```python
from build123d import *

# Parameters (mm, degrees)
SKETCH1_R           = 2.0701
BOSS_EXTRUDE1_DEPTH = 2.286


with BuildPart() as part:
    # Sketch1 → Boss-Extrude1 (new body)
    with BuildSketch(Plane.XY.offset(2.286)):
        with BuildLine():
            Line((-12.7, 3.956428413), (-12.7, -68.893532285))
            Line((-12.7, -68.893532285), (-10.706695129, -69.723))
            Line((-10.706695129, -69.723), (11.870532285, -69.723))
            Line((11.870532285, -69.723), (12.7, -67.729695129))
            Line((12.7, -67.729695129), (12.7, -38.505245425))
            ThreePointArc((12.7, -38.505245425), (14.659980102, -35.571927909), (18.12006403, -36.260181395))
            Line((18.12006403, -36.260181395), (38.820161129, -56.960278494))
            Line((38.820161129, -56.960278494), (40.813466, -57.789746209))
            Line((40.813466, -57.789746209), (56.780673371, -41.822538838))
            Line((56.780673371, -41.822538838), (57.610141086, -39.829233967))
            Line((57.610141086, -39.829233967), (6.081013492, 11.699893628))
            Line((6.081013492, 11.699893628), (4.087708621, 12.529361343))
            Line((4.087708621, 12.529361343), (-11.870532285, 5.949733284))
            Line((-11.870532285, 5.949733284), (-12.7, 3.956428413))
        make_face()
        with Locations((0, -63.5)):
            Circle(SKETCH1_R, mode=Mode.SUBTRACT)
        with Locations((35.921024484, -35.921024484)):
            Circle(SKETCH1_R, mode=Mode.SUBTRACT)
        with Locations((17.960512242, -17.960512242)):
            Circle(SKETCH1_R, mode=Mode.SUBTRACT)
        with Locations((0, -38.1)):
            Circle(SKETCH1_R, mode=Mode.SUBTRACT)
        with Locations((0, -12.7)):
            Circle(SKETCH1_R, mode=Mode.SUBTRACT)
        Circle(SKETCH1_R, mode=Mode.SUBTRACT)
        with Locations((8.980256121, -8.980256121)):
            Circle(SKETCH1_R, mode=Mode.SUBTRACT)
        with Locations((0, -25.4)):
            Circle(SKETCH1_R, mode=Mode.SUBTRACT)
        with Locations((0, -50.8)):
            Circle(SKETCH1_R, mode=Mode.SUBTRACT)
        with Locations((26.940768363, -26.940768363)):
            Circle(SKETCH1_R, mode=Mode.SUBTRACT)
        with Locations((44.901280605, -44.901280605)):
            Circle(SKETCH1_R, mode=Mode.SUBTRACT)
    extrude(amount=-BOSS_EXTRUDE1_DEPTH)


solid = part.part
```
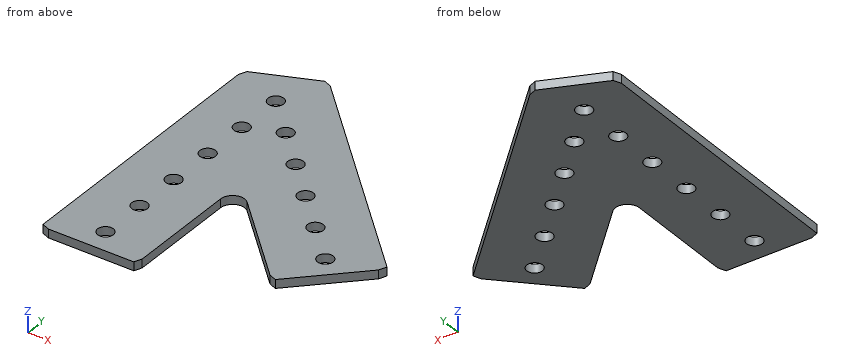
Can you work these out from the model? Positions are in its coordinate system, mm. Give positions to 0.01 mm unless a question says otherwise; leave off trailing zeros. Write each loop counter-clockwise with the first axis right and the second up, starting at its lowest first coordinate (ties: lowest second). Pieces come first, ordered by that corner, then holes. Notation, with made-up numbers: (71.5, -8) - (106.5, -8) arc R18 ccw to (106.5, 11) - close; hole circle Ø9 at (33, -39.5). An arc over 180 degrees is marked (long way). Write item = value, one per line. Start each with the question number.
1. Imagine slicing it at C-C (y = -50.8). Please give me the cut outline in (x, z), and give its area (3 significant figures).
2. Imagine slicing it at B-B (x = 0). Please give me the cut outline in (y, z), and give its area (3 significant figures).
3. Imagine slicing it at D-D (z = 1.8). Count the separate pieces of the cut face and the enclosed holes in it, and give its area (3 significant figures).
4. For pin 1 (3.5 mm diameter, centred on x = 0, y = -25.4, fed in from -Z); pin 2 (1 mm diameter, centred on x = 23, z = 1, fed in from -Y), each with a flat end and sliding along its axis, tell me the tip position at first contact or that it passes through.
5. Please list where these lines run through material, in increasing order: line 1 (X direction, y = -46, z = 1.4); line 2 (X direction, y = -44, z = 0.8); line 3 (Y direction, x = 35, z = 0.75).
6. Imagine slicing it at A-A (y = -63.5). Please give me the cut outline in (x, z), and give its area (3 significant figures).
Worked answers:
q1.outline = (-12.7, 0) - (-2.07, 0) - (-2.07, 2.29) - (-12.7, 2.29) - close; (2.07, 0) - (12.7, 0) - (12.7, 2.29) - (2.07, 2.29) - close; (32.66, 0) - (47.8, 0) - (47.8, 2.29) - (32.66, 2.29) - close
q1.area = 83.2 mm2
q2.outline = (-69.72, 0) - (-65.57, 0) - (-65.57, 2.29) - (-69.72, 2.29) - close; (-61.43, 0) - (-52.87, 0) - (-52.87, 2.29) - (-61.43, 2.29) - close; (-48.73, 0) - (-40.17, 0) - (-40.17, 2.29) - (-48.73, 2.29) - close; (-36.03, 0) - (-27.47, 0) - (-27.47, 2.29) - (-36.03, 2.29) - close; (-23.33, 0) - (-14.77, 0) - (-14.77, 2.29) - (-23.33, 2.29) - close; (-10.63, 0) - (-2.07, 0) - (-2.07, 2.29) - (-10.63, 2.29) - close; (2.07, 0) - (10.84, 0) - (10.84, 2.29) - (2.07, 2.29) - close
q2.area = 127 mm2
q3.separate_pieces = 1
q3.enclosed_holes = 11
q3.area = 3,170 mm2
q4.pin_1 = through
q4.pin_2 = -41.64
q5.line_1 = -12.7 to 12.7, 27.86 to 43.15, 46.66 to 52.6
q5.line_2 = -12.7 to 12.7, 25.86 to 43.04, 46.76 to 54.6
q5.line_3 = -53.14 to -37.77, -34.07 to -17.22
q6.outline = (-12.7, 0) - (-2.07, 0) - (-2.07, 2.29) - (-12.7, 2.29) - close; (2.07, 0) - (12.7, 0) - (12.7, 2.29) - (2.07, 2.29) - close
q6.area = 48.6 mm2
